Read the model definition and answer for the solid it produces. Units are mm, in the model's axes. Round coordinates to 2 decimals unless told otherwise and drop trailing zeros. Order: outer loops, then holes, each group sorted by start corner. A loop starts at its lowest first (then second) coordinate and runs counter-clockwise, first axis right, second up. Notation, with made-up numbers: (56, -10) - (112, -10) arc R29 cw to (112, 24) - close; hole circle Ø9 at (-36.5, 57). An arc over 180 degrees is marked (long way). Put each result on its own line as item: value. Start each with the question number.
Q1. Section A-A on y = 9 is taken. Give the vertices of the cut face in (x, z).
Q2. Section C-C on z = 4.2 is taken. Give the vertices of the cut face in (x, y).
Q3. Find the intervals of material crossed by line 1 along X through (y, z) = (9.5, 3.75); line 2 along X through (y, z) = (7, 4.05); line 3 along Y through (x, z) = (125, 3.95), in increasing order. Write a range as from..to.
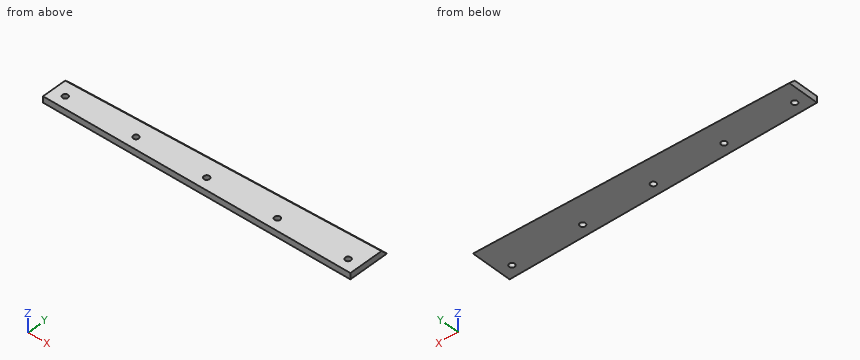
from build123d import *

# Parameters (mm, degrees)
SKETCH1_W            = 5
SKETCH1_H            = 33
BOSS_EXTRUDE1_DEPTH  = 250
CUT_EXTRUDE1_DEPTH   = 253.218159537
CHAMFER1_SIZE        = 5
M4_CLEARANCE_HOLE1_D = 4.5
LPATTERN1_COUNT      = 5
LPATTERN1_PITCH      = 57.5


with BuildPart() as part:
    # Sketch1 → Boss-Extrude1 (new body)
    with BuildSketch(Plane(origin=(0, 0, 0), x_dir=(0, 0, -1), z_dir=(1, 0, 0))):
        with Locations((-2.5, 16.5)):
            Rectangle(SKETCH1_W, SKETCH1_H)
    extrude(amount=BOSS_EXTRUDE1_DEPTH)

    # Sketch2 → Cut-Extrude1 (cut, through all)
    with BuildSketch(Plane.XY):
        Polygon((0, 33), (0, 25), (250, 33), align=None)
    extrude(amount=CUT_EXTRUDE1_DEPTH, mode=Mode.SUBTRACT)

    # Chamfer1
    chamfer1_edges = [part.edges().sort_by_distance(p)[0] for p in [
        (125, 29, 5),
    ]]
    chamfer(chamfer1_edges, length=CHAMFER1_SIZE - 0.0001)  # a hair under: the kernel refuses the full size

    # M4 Clearance Hole1 (through all)
    with Locations(Plane.XY.offset(5)):
        with Locations((240, 9)):
            m4_clearance_hole1 = Hole(M4_CLEARANCE_HOLE1_D / 2)

    # LPattern1: M4 Clearance Hole1 ×5
    with Locations(*[(-i * LPATTERN1_PITCH, 0, 0) for i in range(1, LPATTERN1_COUNT)]):
        add(m4_clearance_hole1, mode=Mode.SUBTRACT)


solid = part.part
Findings:
1. outline: (0, 0) - (7.75, 0) - (7.75, 5) - (0, 5) - close; (12.25, 0) - (65.25, 0) - (65.25, 5) - (12.25, 5) - close; (69.75, 0) - (122.75, 0) - (122.75, 5) - (69.75, 5) - close; (127.25, 0) - (180.25, 0) - (180.25, 5) - (127.25, 5) - close; (184.75, 0) - (237.75, 0) - (237.75, 5) - (184.75, 5) - close; (242.25, 0) - (250, 0) - (250, 5) - (242.25, 5) - close
2. outline: (0, 0) - (250, 0) - (250, 28.8) - (0, 20.8) - close; hole circle Ø4.5 at (10, 9); hole circle Ø4.5 at (67.5, 9); hole circle Ø4.5 at (125, 9); hole circle Ø4.5 at (182.5, 9); hole circle Ø4.5 at (240, 9)
3. line 1: 0..7.81, 12.19..65.31, 69.69..122.81, 127.19..180.31, 184.69..237.81, 242.19..250
3. line 2: 0..8.97, 11.03..66.47, 68.53..123.97, 126.03..181.47, 183.53..238.97, 241.03..250
3. line 3: 0..6.75, 11.25..25.05
